For this review, use the dimensioned drawing (mm, ordinates from the lowest corner) and the shaded views. A direction names the side the tool comes from. Give positions to 0.01 mm unless a question says otherwise; leave off trailing zeros. Order: outer loops, then holes, each group sorted by start corner. A loop starts at its lowest first (then second) coordinate and runs counter-clockwise, first axis right, second up. Notation, with made-up numbers: (47, 2.25) - (62, 2.25) arc R9 cw to (62, 7.25) - close; hole circle Ø9 at (84.5, -24.75). An arc over 180 degrees is marked (long way). Use a Markdown table: item, result. Add a question column.
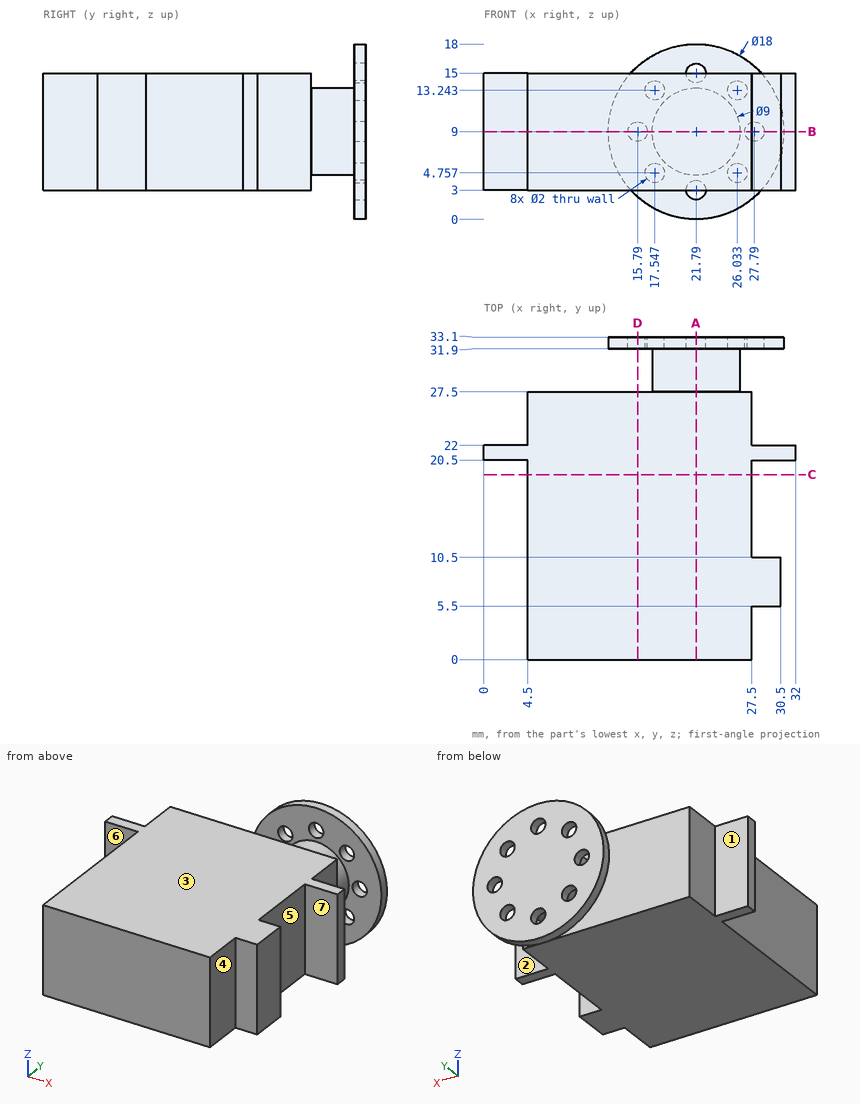
Q1. We need section B-B (z = 9). Count the separate pieces of the cut face and the enclosed holes in it.
Q2. We need section A-A (x = 21.79). Write out the cut boundary in (y, z), plus the area to 3 significant figures.
Q3. Wall thickness on probe 1 along X at (y, z) = (32.5, 9); probe 2 along Y at (x, z) = (20, 14.5); probe 3 along Z at (x, y) = (19, 2): over which ranges is each line inside the solid? List them lowest first.
Q4. Machinability: for the marked faces 1, 2 and 3, which of the approach directions +Z, -Z, +X, -X, +Y, -Y give a long, thin tool a straight path to every point of the face, cutting with its end or side? Answer none if there is none.
Q5. Draft analysis for pull direction Y (two halves, no side actions). For the marked faces 4, 5, 6 and 7, state which applies: pulls with the +Y half, pulls with the -Y half, needs draft (parallel to the pull), parting line crosses it, or undercut.
Q6. We need section D-D (x = 15.79). Write out the cut boundary in (y, z), plus the area to 3 significant figures.
Q7. Clearance check with flat-ended pins moving along their axes: P1, Ø8, axis at y = 7, z = 4, coming from the -X side; P2, Ø5, axis at x = 13, y = 11.5, coming from the +Z side; P3, Ø3, axis at x = 20.5, y = 22, coming from the -Z side; P4, Ø1.6, axis at x = 17.55, z = 4.76, coming from the -Y side. State where each tip first meets the part, or that it passes through.
Q8. We need section C-C (y = 19). Write out the cut boundary in (x, z).
Here are the results:
| question | item | result |
|---|---|---|
| 1 | separate pieces | 3 |
| 1 | enclosed holes | 0 |
| 2 | outline | (0, 3) - (27.5, 3) - (27.5, 4.5) - (31.9, 4.5) - (31.9, 4) - (33.1, 4) - (33.1, 14) - (31.9, 14) - (31.9, 13.5) - (27.5, 13.5) - (27.5, 15) - (0, 15) - close; (31.9, 0) - (33.1, 0) - (33.1, 2) - (31.9, 2) - close; (31.9, 16) - (33.1, 16) - (33.1, 18) - (31.9, 18) - close |
| 2 | area | 386 mm2 |
| 3 | probe 1 | 12.79 to 14.79, 16.79 to 26.79, 28.79 to 30.79 |
| 3 | probe 2 | 0 to 27.5, 31.9 to 33.1 |
| 3 | probe 3 | 3 to 15 |
| 4 | face 1 | +Z, -Z, -X, +Y |
| 4 | face 2 | +Z, -Z, +X |
| 4 | face 3 | +Z, +X, -X, -Y |
| 5 | face 4 | needs draft |
| 5 | face 5 | undercut |
| 5 | face 6 | pulls with the -Y half |
| 5 | face 7 | undercut |
| 6 | outline | (0, 3) - (27.5, 3) - (27.5, 15) - (0, 15) - close; (31.9, 2.29) - (33.1, 2.29) - (33.1, 8) - (31.9, 8) - close; (31.9, 10) - (33.1, 10) - (33.1, 15.71) - (31.9, 15.71) - close |
| 6 | area | 344 mm2 |
| 7 | P1 | x = 4.5 |
| 7 | P2 | z = 15 |
| 7 | P3 | z = 3 |
| 7 | P4 | y = 0 |
| 8 | outline | (4.5, 3) - (27.5, 3) - (27.5, 15) - (4.5, 15) - close |
